from build123d import *

# Parameters (mm, degrees)
SKETCH1_W                               = 110
SKETCH1_H                               = 40
BRACKET_DEPTH                           = 30
CBORE_FOR_M8_HEX_HEAD_BOLT1_D           = 9
CBORE_FOR_M8_HEX_HEAD_BOLT1_CBORE_D     = 18.011
CBORE_FOR_M8_HEX_HEAD_BOLT1_CBORE_DEPTH = 5.3
M6_TAPPED_HOLE1_D                       = 5
M6_TAPPED_HOLE1_DEPTH                   = 10
M6_TAPPED_HOLE1_TIP                     = 1.502151548


with BuildPart() as part:
    # Sketch1 → BRACKET (new body)
    with BuildSketch(Plane.XY):
        Rectangle(SKETCH1_W, SKETCH1_H)
    extrude(amount=BRACKET_DEPTH)

    # CBORE for M8 Hex Head Bolt1 (through all)
    with Locations(Plane.XY.offset(30)):
        with Locations((-40, 0), (-10, 0)):
            CounterBoreHole(CBORE_FOR_M8_HEX_HEAD_BOLT1_D / 2, CBORE_FOR_M8_HEX_HEAD_BOLT1_CBORE_D / 2, CBORE_FOR_M8_HEX_HEAD_BOLT1_CBORE_DEPTH)

    # M6 Tapped Hole1
    with Locations(Plane.XY.offset(30)):
        with Locations((15, 0), (45, 0)):
            Hole(M6_TAPPED_HOLE1_D / 2, depth=M6_TAPPED_HOLE1_DEPTH)
            with Locations((0, 0, -(M6_TAPPED_HOLE1_DEPTH + M6_TAPPED_HOLE1_TIP / 2))):  # 118° drill point
                Cone(0, M6_TAPPED_HOLE1_D / 2, M6_TAPPED_HOLE1_TIP, mode=Mode.SUBTRACT)


solid = part.part
Here's how the part is built. I have some questions about the finished solid (model axes, mm). A direction names the side the tool comes from. Coordinates: 2 decimals unless noted, no trailing zeros. Loops run counter-clockwise (first coordinate to the right, second up) from the corner with the lowest first, then second, coordinate; pieces in that order, holes last.
1. I need wall thicknesses on L1, parallel to Y at x = -10, z = 26.8; L2, parallel to X at y = 4, z = 18.5; L3, parallel to Y at x = 45, z = 22.25. Which ranges of each line are inside material? Lowest first, please.
2. Imagine slicing it at B-B, the plane z = 4. Please give me the cut outline in (x, y).
3. For faces 4 (the flat face through (-55, 0, 15)), 5 (the cylindrical face through (-18.997, 0.396, 27.387)), which set-ups out of +Z, -Z, +X, -X, +Y, -Y let a thin tool reach every point of the face, with its end or its side?
4. Imagine slicing it at A-A, the plane x = -40. Please give me the cut outline in (y, z), and give its area (3 significant figures).
5. If we mould it in two halves opening along Y, with no side actions, what happens to faces 1 (the flat face through (-1, 0, 0)), 2 (the flat face through (-1, 20, 15)), 3 (the cylindrical face through (-44.292, 1.352, 12.177))? For each: pulls with the +Y half, pulls with the -Y half, needs draft (parallel to the pull), parting line crosses it, or undercut.
6. For P1, Ø4, axis at x = 45, y = 0, coming from the +Z side; P2, Ø5.5, axis at x = -43.5, y = 1.5, coming from the +Z side, each with a flat end and sliding along its axis, tell me the tip position at first contact or that it passes through.
Taken from the geometry:
1. L1: y = -20 to -9.01, 9.01 to 20
1. L2: x = -55 to -42.06, -37.94 to -12.06, -7.94 to 55
1. L3: y = -20 to -2.5, 2.5 to 20
2. outline: (-55, -20) - (55, -20) - (55, 20) - (-55, 20) - close; hole circle Ø9 at (-40, 0); hole circle Ø9 at (-10, 0)
3. face 4: +Z, -Z, -X, +Y, -Y
3. face 5: +Z
4. outline: (-20, 0) - (-4.5, 0) - (-4.5, 24.7) - (-9.01, 24.7) - (-9.01, 30) - (-20, 30) - close; (4.5, 0) - (20, 0) - (20, 30) - (9.01, 30) - (9.01, 24.7) - (4.5, 24.7) - close
4. area: 882 mm2
5. face 1: needs draft
5. face 2: pulls with the +Y half
5. face 3: undercut
6. P1: stops at z = 19.7
6. P2: stops at z = 24.7
